Print and shaded views of the part. All mm, measured from the part's lowest x, y and z. A direction names the side the tool comes from. Give positions to 0.01 mm unless a question says otherwise; leave off trailing zeros. Loops run counter-clockwise (first coordinate to the right, second up) from the corner with the lowest first, then second, coordinate; pieces in that order, holes last. Notation, with made-up numbers: M 6,21.5 L 21,21.5 A15 cw 21,42.5 Z; hole C 72,-27.5 d7. An arc over 180 degrees is marked long. Answer in a Markdown table with one row per item.
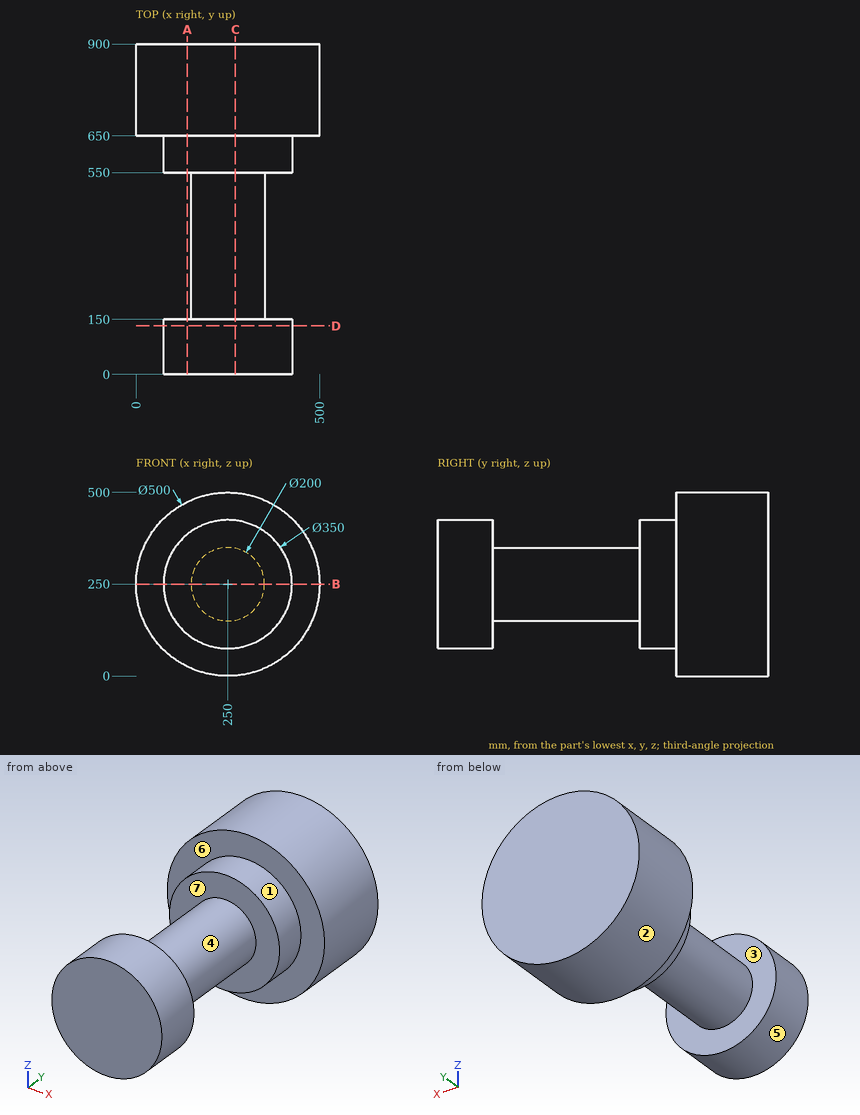
(1) Saw through at D-D, the plane y = 132. Give the cut face in (x, z).
Established:
| item | result |
|---|---|
| outline | C 250,250 d350 |
(2) Wall check: L1, parallel to Y at x = 217, z = 356; L2, parallel to Y at x = 159, z = 42; L3, parallel to Z at x = 52.5, y = 773. Give the ranges that are in metal, low to high.
Established:
| item | result |
|---|---|
| L1 | y = 0 to 150, 550 to 900 |
| L2 | y = 650 to 900 |
| L3 | z = 96.72 to 403.28 |
(3) Mould opens along Y. For the marked faces 4, 5, 6 and 7 say: pulls with the +Y half, pulls with the -Y half, needs draft (parallel to the pull), parting line crosses it, or undercut.
Established:
| item | result |
|---|---|
| face 4 | undercut |
| face 5 | needs draft |
| face 6 | pulls with the -Y half |
| face 7 | undercut |
(4) Which spindle directions (+Z, -Z, +X, -X, +Y, -Y) get a long thin tool onto all of the face, cutting with end or side? Do the marked faces 1, 2 and 3. Say none if no direction does.
Established:
| item | result |
|---|---|
| face 1 | -Y |
| face 2 | +Y, -Y |
| face 3 | none |
(5) Saw through at B-B, the plane z = 250. Give the cut face in (x, y).
Established:
| item | result |
|---|---|
| outline | M 0,650 L 75,650 L 75,550 L 150,550 L 150,150 L 75,150 L 75,0 L 425,0 L 425,150 L 350,150 L 350,550 L 425,550 L 425,650 L 500,650 L 500,900 L 0,900 Z |
(6) Flat gauge pins, fed straight in: P1, Ø3, axis at y = 475.5, z = 239.5, coming from the -X side; P2, Ø1, axis at y = 659.5, z = 316, coming from the +X side; P3, Ø1.5, axis at x = 190, y = 174.5, coming from the -Z side. Where does each tip first touch, or does it go through?
Established:
| item | result |
|---|---|
| P1 | stops at x = 150.41 |
| P2 | stops at x = 491.27 |
| P3 | stops at z = 169.44 |
(7) Saw through at C-C, the plane x = 270.5. Give the cut face in (y, z), and give its area (3 significant figures).
Established:
| item | result |
|---|---|
| outline | M 0,76.2 L 150,76.2 L 150,152.12 L 550,152.12 L 550,76.2 L 650,76.2 L 650,0.84 L 900,0.84 L 900,499.16 L 650,499.16 L 650,423.8 L 550,423.8 L 550,347.88 L 150,347.88 L 150,423.8 L 0,423.8 Z |
| area | 290,000 mm2 |
(8) Saw through at A-A, the plane x = 140. Give the cut face in (y, z).
Established:
| item | result |
|---|---|
| outline | M 0,113.89 L 150,113.89 L 150,386.11 L 0,386.11 Z; M 550,113.89 L 650,113.89 L 650,25.5 L 900,25.5 L 900,474.5 L 650,474.5 L 650,386.11 L 550,386.11 Z |
